The listing builds one solid part. Answer for the finished solid, in the listing's coordinates (mm). Face numbers are marked on the shaded views. A direction names the side the tool comes from. Give positions to 0.01 mm unless a question says otherwise; leave off trailing zeros. Write each loop counter-clockwise with the first axis right and the second up, starting at its lowest first coordinate (ties: lowest second). Pieces come first, ordered by that corner, then holes. Notation, with made-up numbers: M 76.5,-14 L 125.5,-14 A6 cw 125.5,-9 Z; hole C 24.25,78 d4. An arc over 180 degrees is marked long. Return JSON: item names as keys, results as strings.
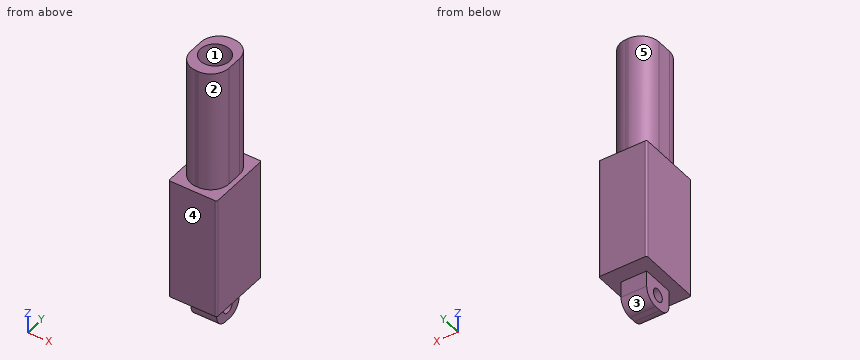
from build123d import *

# Parameters (mm, degrees)
SKETCH_1_W          = 15
SKETCH_1_H          = 20
EXTRUDE_1_DEPTH     = 38
EXTRUDE_2_DEPTH     = 38
SKETCH_3_W          = 8
SKETCH_3_H          = 10
EXTRUDE_3_DEPTH     = 9
FILLET_1_R          = 4
SKETCH_4_R          = 2
CUT_EXTRUDE_1_DEPTH = 78.512902152
FILLET_2_R          = 0.5
SKETCH_5_R          = 4.5
CUT_EXTRUDE_2_DEPTH = 35


with BuildPart() as part:
    # Эскиз1 → Бобышка-Вытянуть1 (new body)
    with BuildSketch(Plane.XY):
        Rectangle(SKETCH_1_W, SKETCH_1_H)
    extrude(amount=EXTRUDE_1_DEPTH)

    # Эскиз2 → Бобышка-Вытянуть2 (add)
    with BuildSketch(Plane.XY.offset(38)):
        with BuildLine():
            Line((0.3, -8), (-0.3, -8))
            ThreePointArc((-0.3, -8), (-4.330508653, -6.330508653), (-6, -2.3))
            Line((-6, -2.3), (-6, 2.3))
            ThreePointArc((-6, 2.3), (-4.330508653, 6.330508653), (-0.3, 8))
            Line((-0.3, 8), (0.3, 8))
            ThreePointArc((0.3, 8), (4.330508653, 6.330508653), (6, 2.3))
            Line((6, 2.3), (6, -2.3))
            ThreePointArc((6, -2.3), (4.330508653, -6.330508653), (0.3, -8))
        make_face()
    extrude(amount=EXTRUDE_2_DEPTH)

    # Эскиз3 → Бобышка-Вытянуть3 (add)
    with BuildSketch(Plane(origin=(0, 0, 0), x_dir=(-1, 0, 0), z_dir=(0, 0, -1))):
        Rectangle(SKETCH_3_W, SKETCH_3_H)
    extrude(amount=EXTRUDE_3_DEPTH)

    # Скругление1
    fillet_1_edges = [part.edges().sort_by_distance(p)[0] for p in [
        (0, 5, -9),
        (0, -5, -9),
    ]]
    fillet(fillet_1_edges, radius=FILLET_1_R)

    # Эскиз4 → Вырез-Вытянуть1 (cut, through all)
    with BuildSketch(Plane.ZY.offset(4)):
        with Locations((-4.7, 0)):
            Circle(SKETCH_4_R)
    extrude(amount=-CUT_EXTRUDE_1_DEPTH, mode=Mode.SUBTRACT)

    # Скругление2
    fillet_2_edges = [part.edges().sort_by_distance(p)[0] for p in [
        (-7.5, 10, 19),
        (7.5, 10, 19),
        (7.5, -10, 19),
        (-7.5, -10, 19),
    ]]
    fillet(fillet_2_edges, radius=FILLET_2_R)

    # Эскиз5 → Вырез-Вытянуть2 (cut)
    with BuildSketch(Plane.XY.offset(76)):
        Circle(SKETCH_5_R)
    extrude(amount=-CUT_EXTRUDE_2_DEPTH, mode=Mode.SUBTRACT)


solid = part.part
Item 1: A cutting plane is placed at A-A, the plane y = 0. Write down the section's boundary in (x, z), plus the area to 3 significant figures.
Geometry results:
{"outline": "M -7.5,0 L -4,0 L -4,-2.7 L 4,-2.7 L 4,0 L 7.5,0 L 7.5,38 L 6,38 L 6,76 L 4.5,76 L 4.5,41 L -4.5,41 L -4.5,76 L -6,76 L -6,38 L -7.5,38 Z; M -4,-9 L 4,-9 L 4,-6.7 L -4,-6.7 Z", "area": "751 mm2"}
Item 2: Find the intervals of material crossed by line 1 (Y direction, x = 0, z = -4.7); line 2 (Y direction, x = 0, z = 64); line 3 (X direction, y = 2.75, z = 65), in increasing order.
Geometry results:
{"line 1": "y = -5 to -2, 2 to 5", "line 2": "y = -8 to -4.5, 4.5 to 8", "line 3": "x = -5.98 to -3.56, 3.56 to 5.98"}
Item 3: A cutting plane is placed at C-C, the plane x = 3. Write down the section's boundary in (y, z).
Geometry results:
{"outline": "M -10,0 L -5,0 L -5,-5 A4 ccw -1,-9 L 1,-9 A4 ccw 5,-5 L 5,0 L 10,0 L 10,38 L 7.32,38 L 7.32,76 L 3.35,76 L 3.35,41 L -3.35,41 L -3.35,76 L -7.32,76 L -7.32,38 L -10,38 Z; hole C 0,-4.7 d4"}
Item 4: Which of the six approach directions +Z, -Z, +X, -X, +Y, -Y give full straight-line access (tool end or side, diameter ignored) to the marked faces 4 and 5?
Geometry results:
{"face 4": "+Z, -Z, +X, -X, -Y", "face 5": "+Z, -X, +Y"}
Item 5: Determine the mould class of the marked faces 1, 2 and 3 for opening direction X: +X half, -X half, draft (parallel to the pull), parting line (faces both ways), or undercut.
Geometry results:
{"face 1": "undercut", "face 2": "+X half", "face 3": "draft"}
Item 6: A cutting plane is placed at D-D, the plane y = 6.5. Write down the section's boundary in (x, z).
Geometry results:
{"outline": "M -7.5,0 L 7.5,0 L 7.5,38 L 4.15,38 L 4.15,76 L -4.15,76 L -4.15,38 L -7.5,38 Z"}
Item 7: A cutting plane is placed at B-B, the plane z = 44.5. Write down the section's boundary in (x, y).
Geometry results:
{"outline": "M -6,-2.3 A5.7 ccw -0.3,-8 L 0.3,-8 A5.7 ccw 6,-2.3 L 6,2.3 A5.7 ccw 0.3,8 L -0.3,8 A5.7 ccw -6,2.3 Z; hole C 0,0 d9"}
Item 8: Given pin 1 Ø2 at (x, z) = (1.5, 65.5) entering from +Y; pin 2 Ø5.5 at (x, z) = (0.5, -3) entering from +Y; pin 3 Ø5.5 at (x, z) = (-1.5, -3.5) entering from -Y, each flat-ended and moving along its own axis, determine where each tip first touches the part or whether it passes through.
Geometry results:
{"pin 1": "stops at y = 8", "pin 2": "stops at y = 5", "pin 3": "stops at y = -5"}
